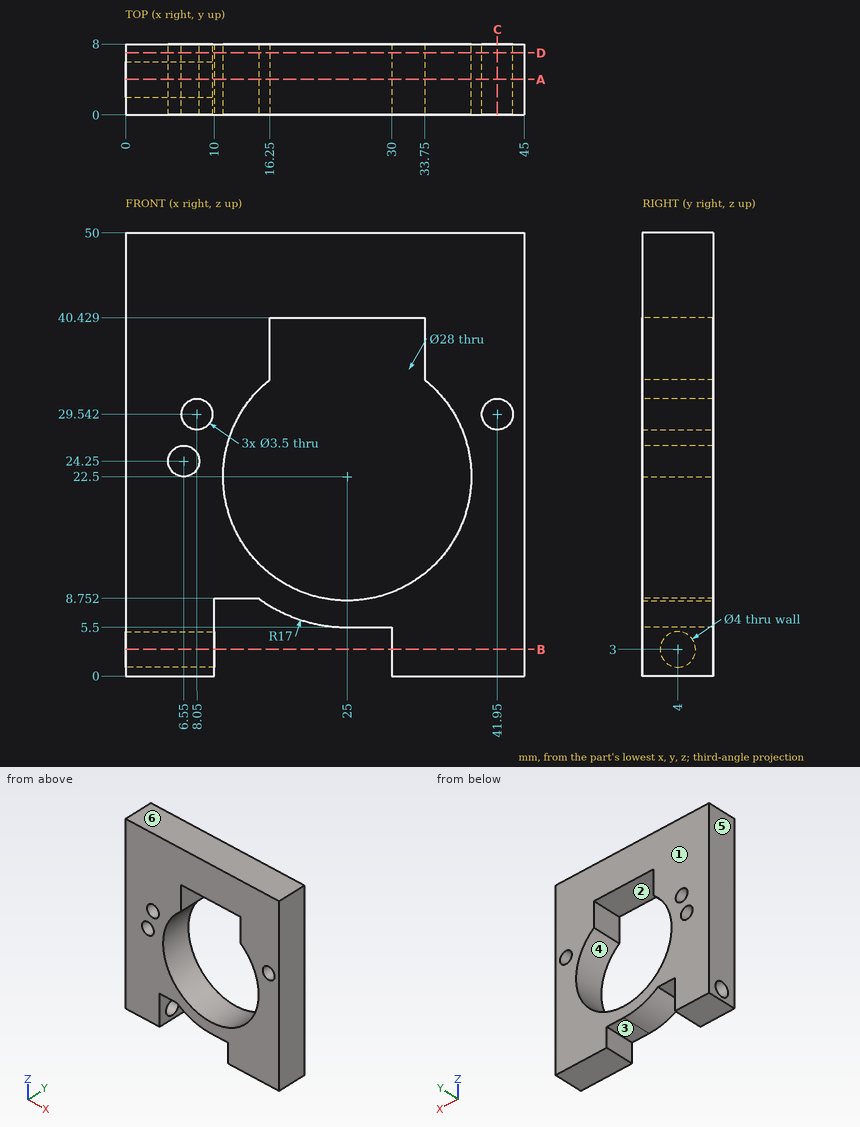
The figure shows three views and two pictorial views of one solid part (mm, origin at its lowest corner). Answer the questions. A direction names the side the tool comes from. Give positions to 0.01 mm unless a question says otherwise; leave off trailing zeros. Order: outer loops, then holes, each group sorted by start corner. A loop starts at its lowest first (then second) coordinate and runs counter-clockwise, first axis right, second up. Notation, with made-up numbers: M -5.75,89.25 L 12.25,89.25 A19 cw 12.25,104.25 Z; hole C 84,66.25 d1. An arc over 180 degrees is marked long. Return JSON: item names as keys, results as strings.
Q1. Find section B-B, the plane z = 3. Write down the section's boundary in (x, y).
Answer below:
{"outline": "M 0,0 L 10,0 L 10,2 L 0,2 Z; M 0,6 L 10,6 L 10,8 L 0,8 Z; M 30,0 L 45,0 L 45,8 L 30,8 Z"}
Q2. Each of these flat-tipped pins is pushed along its axis until it touches: pin 1 (2.5 mm diameter, centred on x = 27, y = 2.5, fed in from -Z); pin 2 (1.6 mm diameter, centred on y = 3, z = 3.5, fed in from -X); pin 3 (1.5 mm diameter, centred on x = 12, y = 4.5, fed in from -Z). Where does it stop, or does it pass through?
Answer below:
{"pin 1": "stops at z = 5.5", "pin 2": "stops at x = 30", "pin 3": "stops at z = 8.75"}
Q3. Which of the six approach directions +Z, -Z, +X, -X, +Y, -Y give full straight-line access (tool end or side, diameter ignored) to the marked faces 1, 2 and 3?
Answer below:
{"face 1": "+Z, -Z, +X, -X, +Y", "face 2": "+Y, -Y", "face 3": "-Z, +Y, -Y"}
Q4. The mould has two halves that part along X. Classify the marked faces 4, 5 and 6: pulls with the +X half, pulls with the -X half, needs draft (parallel to the pull), parting line crosses it, or undercut.
Answer below:
{"face 4": "undercut", "face 5": "pulls with the -X half", "face 6": "needs draft"}
Q5. Find section D-D, the plane y = 7. Write down the section's boundary in (x, z).
Answer below:
{"outline": "M 0,0 L 10,0 L 10,8.75 L 15,8.75 A17 ccw 25,5.5 L 30,5.5 L 30,0 L 45,0 L 45,50 L 0,50 Z; hole C 6.55,24.25 d3.5; hole C 8.05,29.54 d3.5; hole M 16.25,33.43 A14 ccw long 33.75,33.43 L 33.75,40.43 L 16.25,40.43 Z; hole C 41.95,29.54 d3.5"}
Q6. Find the intervals of material crossed by line 1 along Z through (x, y) = (41.95, 5.5); line 2 along Y through (x, z) = (3, 3); line 3 along X through (y, z) = (4.5, 39), in increasing order. Write a range as [from, to].
Answer below:
{"line 1": "z = [0, 27.79], [31.29, 50]", "line 2": "y = [0, 2], [6, 8]", "line 3": "x = [0, 16.25], [33.75, 45]"}
Q7. Find section A-A, the plane y = 4. Write down the section's boundary in (x, z).
Answer below:
{"outline": "M 0,0 L 10,0 L 10,1 L 0,1 Z; M 0,5 L 10,5 L 10,8.75 L 15,8.75 A17 ccw 25,5.5 L 30,5.5 L 30,0 L 45,0 L 45,50 L 0,50 Z; hole C 6.55,24.25 d3.5; hole C 8.05,29.54 d3.5; hole M 16.25,33.43 A14 ccw long 33.75,33.43 L 33.75,40.43 L 16.25,40.43 Z; hole C 41.95,29.54 d3.5"}
Q8. Find section C-C, the plane x = 41.95. Write down the section's boundary in (y, z).
Answer below:
{"outline": "M 0,0 L 8,0 L 8,27.79 L 0,27.79 Z; M 0,31.29 L 8,31.29 L 8,50 L 0,50 Z"}
